Check sheet for the modelled part. Datum: model origin and axes. Units: mm. Face numbers are marked on the shaded views. A direction names the side the tool comes from. Give positions to 0.01 mm unless a question says otherwise; leave off trailing zeros. Order: outer loops, then holes, each group sorted by start corner. A loop starts at its lowest first (then second) coordinate and runs counter-clockwise, first axis right, second up.
Item 1: Gauge pin test, flat ends, axial feed: P1, Ø2, axis at y = 139, z = 161.5, coming from the -X side; P2, Ø1.5, axis at x = 136.5, z = 168, coming from the +Y side; P3, Ø2, axis at y = 133, z = 171.5, coming from the +X side. Record the tip position at first contact, or that the pin passes through.
Item 2: Sectioned sample at A-A on y = 133.5. Record the boundary of the cut face in (x, z), and give its area (3 significant figures).
Item 3: Sectioned sample at D-D on x = 132.75. Record the boundary of the cut face in (y, z), and give its area (3 significant figures).
Item 4: Release check for a two-part mould opening along Z. For the marked faces 1, 2, 3 and 4 record: released by +Z, released by -Z, zero draft, split by the parting line, or undercut.
Item 5: Sectioned sample at B-B on x = 137.5. Record the boundary of the cut face in (y, z).
Item 6: Material ranges on line 1 along Z through (x, y) = (142.75, 136); line 2 along Y through (x, z) = (139.25, 158.25); line 3 along X through (y, z) = (140, 153), recorded low to high.
Item 7: Access from +Z, -Z, +X, -X, +Y, -Y to the whole of each face (thin tool, end or side, straight path). Record for the marked faces 5 and 6.
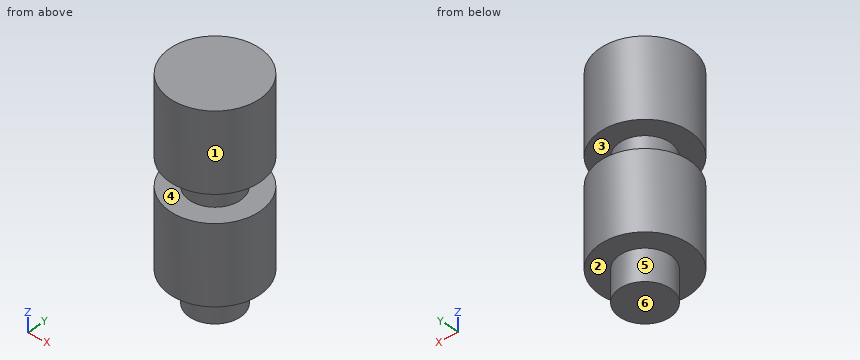
from build123d import *

# Parameters (mm, degrees)
CYLINDER037_R     = 5.75
CYLINDER037_DEPTH = 10
CYLINDER036_R     = 3.25
CYLINDER036_DEPTH = 10
CYLINDER035_R     = 5.75
CYLINDER035_DEPTH = 10
CYLINDER034_R     = 3.25
CYLINDER034_DEPTH = 10


with BuildPart() as obj1:
    # Cylinder037 → Cylinder037 (new body)
    with BuildSketch(Plane(origin=(-23, 0, 69), x_dir=(1, 0, 0), z_dir=(0, 0, 1))):
        Circle(CYLINDER037_R)
    extrude(amount=CYLINDER037_DEPTH)


with BuildPart() as fusion012:
    # Cylinder036 → Cylinder036 (new body)
    with BuildSketch(Plane(origin=(-23, 0, 65), x_dir=(1, 0, 0), z_dir=(0, 0, 1))):
        Circle(CYLINDER036_R)
    extrude(amount=CYLINDER036_DEPTH)

    # Fusion012: union obj1
    add(obj1.part)


with BuildPart() as fusion012_1:
    # Fusion012 placement: moved
    add(fusion012.part.moved(Location((2.5, -25, -19.5))))


with BuildPart() as obj2:
    # Cylinder035 → Cylinder035 (new body)
    with BuildSketch(Plane(origin=(-23, 0, 69), x_dir=(1, 0, 0), z_dir=(0, 0, 1))):
        Circle(CYLINDER035_R)
    extrude(amount=CYLINDER035_DEPTH)


with BuildPart() as antennacuts001:
    # Cylinder034 → Cylinder034 (new body)
    with BuildSketch(Plane(origin=(-23, 0, 65), x_dir=(1, 0, 0), z_dir=(0, 0, 1))):
        Circle(CYLINDER034_R)
    extrude(amount=CYLINDER034_DEPTH)

    # Fusion011: union obj2
    add(obj2.part)


with BuildPart() as antennacuts001_1:
    # Fusion011 placement: moved
    add(antennacuts001.part.moved(Location((2.5, -25, -6))))

    # Fusion013: union Fusion012
    add(fusion012_1.part)


with BuildPart() as antennacuts001_2:
    # Fusion013 placement: moved
    add(antennacuts001_1.part.moved(Location((158, 162.5, 105))))


solid = antennacuts001_2.part
Report:
1. P1: stops at x = 131.77
1. P2: stops at y = 143.24
1. P3: stops at x = 142.06
2. outline: (133.37, 154.5) - (141.63, 154.5) - (141.63, 164.5) - (133.37, 164.5) - close; (133.37, 168) - (141.63, 168) - (141.63, 178) - (133.37, 178) - close
2. area: 165 mm2
3. outline: (134.26, 154.5) - (140.74, 154.5) - (140.74, 164.5) - (134.26, 164.5) - close; (134.26, 168) - (140.74, 168) - (140.74, 178) - (134.26, 178) - close
3. area: 130 mm2
4. face 1: zero draft
4. face 2: released by -Z
4. face 3: undercut
4. face 4: undercut
5. outline: (131.75, 154.5) - (134.25, 154.5) - (134.25, 150.5) - (140.75, 150.5) - (140.75, 154.5) - (143.25, 154.5) - (143.25, 164.5) - (140.75, 164.5) - (140.75, 168) - (143.25, 168) - (143.25, 178) - (131.75, 178) - (131.75, 168) - (134.25, 168) - (134.25, 164.5) - (131.75, 164.5) - close
6. line 1: z = 154.5 to 164.5, 168 to 178
6. line 2: y = 132.02 to 142.98
6. line 3: x = 135.42 to 139.58
7. face 5: -Z
7. face 6: -Z, +X, -X, +Y, -Y
